Read the model definition and answer for the solid it produces. Units are mm, in the model's axes. Face numbers are marked on the shaded views. A direction names the side the tool comes from. Coordinates: 2 decimals unless noted, no trailing zeros. Order: outer loops, then holes, each group sorted by start corner. A loop starts at its lowest first (then second) coordinate and runs counter-clockwise, first axis right, second up. Notation, with made-up numbers: (-18, -19.5) -> (36, -19.5) arc R21 ccw to (36, 3.5) -> close; hole circle Ø8 at (21, 73.25). An arc over 180 degrees is marked (long way). Use CSV: the item, a comma, the result in double quotes.
```python
from build123d import *

# Parameters (mm, degrees)
SKETCH2_W           = 120
SKETCH2_H           = 100
BOSS_EXTRUDE2_DEPTH = 65
SKETCH3_W           = 100
SKETCH3_H           = 85
CUT_EXTRUDE1_DEPTH  = 55
SKETCH6_R           = 9
SKETCH6_R_2         = 4.9
CUT_EXTRUDE3_DEPTH  = 30
SKETCH8_W           = 4.7
SKETCH8_H           = 4
SKETCH8_H_2         = 5
CUT_EXTRUDE6_DEPTH  = 95
SKETCH9_W           = 5
SKETCH9_H           = 65
CUT_EXTRUDE7_DEPTH  = 4.7
SKETCH10_W          = 82.5
SKETCH10_H          = 54
CUT_EXTRUDE9_DEPTH  = 10


with BuildPart() as part:
    # Sketch2 → Boss-Extrude2 (new body)
    with BuildSketch(Plane(origin=(0, 0, 0), x_dir=(1, 0, 0), z_dir=(0, 1, 0))):
        Rectangle(SKETCH2_W, SKETCH2_H)
    extrude(amount=BOSS_EXTRUDE2_DEPTH)

    # Sketch3 → Cut-Extrude1 (cut)
    with BuildSketch(Plane(origin=(0, 65, 0), x_dir=(1, 0, 0), z_dir=(0, 1, 0))):
        Rectangle(SKETCH3_W, SKETCH3_H)
    extrude(amount=-CUT_EXTRUDE1_DEPTH, mode=Mode.SUBTRACT)

    # Sketch6 → Cut-Extrude3 (cut)
    with BuildSketch(Plane.XY.offset(-42.5)):
        with Locations((0, 50)):
            Circle(SKETCH6_R)
        with Locations((0, 20)):
            Circle(SKETCH6_R_2)
    extrude(amount=-CUT_EXTRUDE3_DEPTH, mode=Mode.SUBTRACT)

    # Sketch8 → Cut-Extrude6 (cut)
    with BuildSketch(Plane.XY.offset(50)):
        with Locations((57.65, 2)):
            Rectangle(SKETCH8_W, SKETCH8_H)
        with Locations((57.65, 62.5)):
            Rectangle(SKETCH8_W, SKETCH8_H_2)
    extrude(amount=-CUT_EXTRUDE6_DEPTH, mode=Mode.SUBTRACT)

    # Sketch9 → Cut-Extrude7 (cut)
    with BuildSketch(Plane(origin=(60, 0, 0), x_dir=(0, 0, -1), z_dir=(1, 0, 0))):
        with Locations((47.5, 32.5)):
            Rectangle(SKETCH9_W, SKETCH9_H)
    extrude(amount=-CUT_EXTRUDE7_DEPTH, mode=Mode.SUBTRACT)

    # Sketch10 → Cut-Extrude9 (cut)
    with BuildSketch(Plane(origin=(60, 0, 0), x_dir=(0, 0, -1), z_dir=(1, 0, 0))):
        with Locations((1.25, 31.5)):
            Rectangle(SKETCH10_W, SKETCH10_H)
    extrude(amount=-CUT_EXTRUDE9_DEPTH, mode=Mode.SUBTRACT)


solid = part.part
```
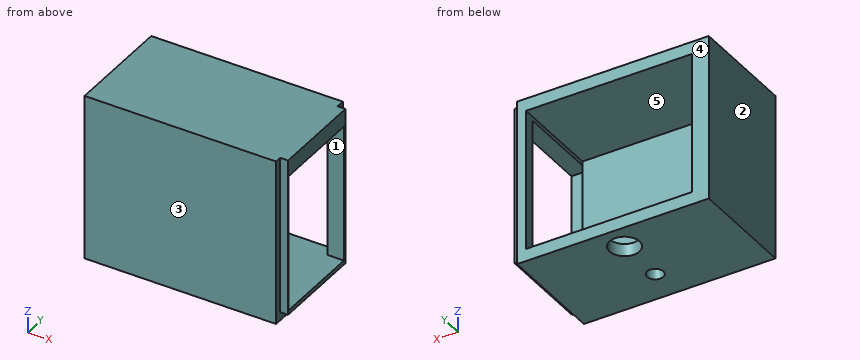
Item 1: Find section C-C, the plane z = -29. Give the vertices of the cut face in (x, y), then the cut area to 3 significant figures.
Return value:
outline,"(-60, 0) -> (55.3, 0) -> (55.3, 4) -> (60, 4) -> (60, 4.5) -> (50, 4.5) -> (50, 10) -> (-50, 10) -> (-50, 65) -> (-60, 65) -> close; (50, 58.5) -> (60, 58.5) -> (60, 60) -> (55.3, 60) -> (55.3, 65) -> (50, 65) -> close"
area,"1,720 mm^2"
Item 2: A tool of negligible diameter and unlimited length cuts with its end or side. For the marked faces 4 and 5, from which of +Z, -Z, +X, -X, +Y, -Y can it reach the whole face along a straight path? Write none if from no direction.
Return value:
face 4,"+Z, -Z, +X, -X, +Y"
face 5,"+Y"
Item 3: Find section D-D, the plane x = -28. Give the vertices of the cut face in (y, z).
Return value:
outline,"(0, -50) -> (65, -50) -> (65, -42.5) -> (10, -42.5) -> (10, 42.5) -> (65, 42.5) -> (65, 50) -> (0, 50) -> close"
Item 4: Find section A-A, the plane x = 0. Give the vertices of the cut face in (y, z), then the cut area to 3 significant figures.
Return value:
outline,"(0, -50) -> (15.1, -50) -> (15.1, -42.5) -> (10, -42.5) -> (10, 42.5) -> (65, 42.5) -> (65, 50) -> (0, 50) -> close; (24.9, -50) -> (41, -50) -> (41, -42.5) -> (24.9, -42.5) -> close; (59, -50) -> (65, -50) -> (65, -42.5) -> (59, -42.5) -> close"
area,"1,620 mm^2"
Item 5: The mould has two halves that part along Y. Classify the marked faces 1, 2 and 3: +Y half, -Y half, draft (parallel to the pull), parting line (faces both ways), or undercut.
Return value:
face 1,"undercut"
face 2,"draft"
face 3,"-Y half"
Item 6: Straight lines are drawn through the part: line 1 along Y through (x, z) = (0, -44.5); line 2 along Z through (x, y) = (-20, 43.5); line 3 along X through (y, z) = (61, -32). For each, find the intervals that lie inside material, in ascending order.
Return value:
line 1,"y = 0 to 15.1, 24.9 to 41, 59 to 65"
line 2,"z = -50 to -42.5, 42.5 to 50"
line 3,"x = -60 to -50, 50 to 55.3"
Item 7: Each of these flat-tipped pins is pushed along its axis until it touches: P1, Ø2.5, axis at x = 58, z = -6, coming from the +Y side; P2, Ø1.6, axis at y = 7.5, z = -13.5, coming from the +X side; P3, Ø2.5, axis at x = 57.5, z = 16, coming from the -Y side. Where does it stop, or does it pass through?
Return value:
P1,"stops at y = 60"
P2,"stops at x = 50"
P3,"stops at y = 4"
Item 8: Find section B-B, the plane y = 50. Give the vertices of the cut face in (x, z).
Return value:
outline,"(-60, -50) -> (-9, -50) -> (-9, -42.5) -> (-50, -42.5) -> (-50, 42.5) -> (50, 42.5) -> (50, 40) -> (60, 40) -> (60, 50) -> (-60, 50) -> close; (9, -50) -> (55.3, -50) -> (55.3, -45) -> (60, -45) -> (60, -42.5) -> (9, -42.5) -> close"
